Could you check a few things on this model? Use its own coordinates, in mm. A direction names the side the tool comes from. Coordinates: 2 decimals unless noted, no trailing zeros. Order: outer loops, then holes, each group sorted by start corner. A loop starts at its lowest first (then second) coordinate and runs counter-clockwise, first axis right, second up. Notation, with made-up numbers: (58, 53) -> (97, 53) arc R18 cw to (97, 84) -> close; hole circle Ø4 at (0, -14). An arc over 180 degrees is marked (long way). Return JSON: item names as keys, results as strings. Group by question number.
Autodesk Inventor part; units mm, degrees
ref_plane "YZ Plane" through (0, 0, 0) normal (1, 0, 0) x (0, 1, 0)
ref_plane "XZ Plane" through (0, 0, 0) normal (0, 1, 0) x (-1, 0, 0)
ref_plane "XY Plane" through (0, 0, 0) normal (0, 0, 1) x (1, 0, 0)
sketch "Sketch1" plane through (0, 0, 0) normal (0, 0, 1) x (1, 0, 0)
  line L0 (-20, 22.5) -> (20, 22.5)
  line L1 (20, 22.5) -> (20, -100)
  line L2 (20, -100) -> (-20, -100)
  line L3 (-20, -100) -> (-20, 22.5)
  circle A0 centre (0, 0) radius 2.5
  dimension "d0" = 122.5
  dimension "d1" = 40
  dimension "d2" = 20
  dimension "d3" = 22.5
  dimension "d4" = 5
extrude "Extrusion1" add sketch "Sketch1" along normal blind 5
sketch "Sketch2" plane through (0, 0, 5) normal (0, 0, 1) x (1, 0, 0)
  line L0 (20, 22.5) -> (-20, 22.5)
  line L1 (-20, -100) -> (20, -100)
  line L2 (-20, 22.5) -> (20, 22.5)
  line L3 (20, 22.5) -> (20, -100)
  line L4 (20, -100) -> (-20, -100)
  line L5 (-20, -100) -> (-20, 22.5)
  line L6 (15, -95) -> (-15, -95)
  line L7 (-15, -95) -> (-15, 17.5)
  line L8 (-15, 17.5) -> (15, 17.5)
  line L9 (15, 17.5) -> (15, -95)
  point P0 (0, 0)
  dimension "d7" = 5
  dimension "d8" = 5
  dimension "d9" = 5
  dimension "d10" = 5
extrude "Extrusion2" add sketch "Sketch2" along normal blind 35
sketch "Sketch3" plane through (-20, -100, 0) normal (0, -1, 0) x (1, 0, 0)
  circle A0 centre (20, 20) radius 8.5
  line L0 (40, 0) -> (40, 40)
  line L1 (0, 0) -> (40, 0)
  circle A1 centre (20, 11.5) radius 1.5
  circle A2 centre (20, 28.5) radius 1.5
  circle A3 centre (20, 20) radius 3.75
  line L2 (0, 0) -> (0, 40)
  point P0 (20, 0)
  dimension "d13" = 20
  dimension "d14" = 20
  dimension "d15" = 17
  dimension "d16" = 3
  dimension "d17" = 7.5
  dimension "d18" = 3
  dimension "d19" = 20
  dimension "d20" = 20
sketch "Sketch4" plane through (0, 0, 5) normal (0, 0, 1) x (1, 0, 0)
  line L0 (-15, 17.5) -> (-15, -95)
  line L1 (15, 17.5) -> (15, -95)
  line L2 (-15, 17.5) -> (15, 17.5)
  line L3 (15, 17.5) -> (15, -17.5)
  line L4 (15, -17.5) -> (-15, -17.5)
  line L5 (-15, -17.5) -> (-15, 17.5)
  point P0 (0, 0)
  point P1 (-15, -17.5)
  dimension "d21" = 35
extrude "Extrusion3" add sketch "Sketch4" along normal blind 20
sketch "Sketch5" plane through (0, 0, 0) normal (0, 0, -1) x (-1, 0, 0)
  circle A0 centre (0, 0) radius 2.5
  circle A1 centre (0, 0) radius 9.5
  dimension "d24" = 19
extrude "Extrusion4" cut sketch "Sketch5" against normal blind 12.5 contours A0 | A1
sketch "Sketch6" plane through (0, 0, 0) normal (0, 0, -1) x (-1, 0, 0)
  circle A0 centre (0, 0) radius 11.5
  dimension "d27" = 23
extrude "Extrusion5" cut sketch "Sketch6" against normal blind 6.5
fillet "Fillet1" radius 2 2 edges at (-20, 22.5, 20) (20, 22.5, 20)
sketch "Sketch7" plane through (0, 0, 0) normal (0, 0, -1) x (-1, 0, 0)
  circle A0 centre (0, 0) radius 6.2
  circle A1 centre (0, 6.2) radius 1.45
  line L0 (0, 6.2) -> (0, 0)
  line L1 (0, 0) -> (6.4707, -3.7359)
  line L2 (0, 0) -> (-6.6791, -3.8562)
  circle A2 centre (5.3694, -3.1) radius 1.45
  circle A3 centre (-5.3694, -3.1) radius 1.45
  dimension "d31" = 12.4
  dimension "d32" = 120
  dimension "d33" = 120
  dimension "d34" = 2.9
  dimension "d35" = 2.9
  dimension "d36" = 2.9
extrude "Extrusion6" cut sketch "Sketch7" against normal blind 25 contours A1 L0 A0 | A0 A1 | A2 A0 | A0 L1 A2 | L0 A1 A0 | A0 A2 L1 | A3 L2 A0 | A0 L2 A3 | A3 A0 L2 | A3 L2 A0
sketch "Sketch8" plane through (0, 0, 25) normal (0, 0, 1) x (1, 0, 0)
  circle A0 centre (5.3694, -3.1) radius 1.45
  circle A1 centre (5.3694, -3.1) radius 4
  circle A2 centre (-5.3694, -3.1) radius 1.45
  circle A3 centre (-5.3694, -3.1) radius 4
  circle A4 centre (0, 6.2) radius 1.45
  circle A5 centre (0, 6.2) radius 4
  point P0 (0, 0)
  dimension "d39" = 8
  dimension "d40" = 8
  dimension "d41" = 8
extrude "Extrusion7" cut sketch "Sketch8" against normal blind 7
fillet "Fillet2" radius 2 3 edges at (0, -17.5, 5) (-15, -56.25, 5) (15, -56.25, 5)
sketch "Sketch9" plane through (0, 0, 40) normal (0, 0, 1) x (1, 0, 0)
  line L0 (20, -100) -> (20, 20.5)
  line L1 (-20, 20.5) -> (-20, -100)
  line L2 (20, -100) -> (-20, -100)
  line L3 (-20, -100) -> (-20, -60)
  line L4 (-20, -60) -> (20, -60)
  line L5 (20, -60) -> (20, -100)
  line L6 (0, -60) -> (-20, -60)
  line L7 (-20, -60) -> (-20, -100)
  line L8 (-20, -100) -> (0, -100)
  line L9 (0, -100) -> (0, -60)
  line L10 (15, -95) -> (-15, -95)
  line L11 (15, -65) -> (-15, -65)
  line L12 (-15, -65) -> (-15, -95)
  line L13 (-15, -95) -> (15, -95)
  line L14 (15, -95) -> (15, -65)
  point P0 (0, 0)
  dimension "d45" = 40
  dimension "d46" = 5
  dimension "d47" = 5
extrude "Extrusion8" add sketch "Sketch9" along normal blind 60 contours L2 L9 L10 L14 L11 L4 L0 | L2 L1 L4 L9 L11 L12 L10
sketch "Sketch10" plane through (0, 0, 100) normal (0, 0, 1) x (1, 0, 0)
  line L0 (-20, -100) -> (20, -100)
  line L1 (20, -100) -> (20, 20.5)
  line L2 (-20, -100) -> (20, -100)
  line L3 (20, -100) -> (20, -60)
  line L4 (20, -60) -> (-20, -60)
  line L5 (-20, -60) -> (-20, -100)
  point P0 (0, 0)
  dimension "d50" = 40
extrude "Extrusion9" add sketch "Sketch10" against normal blind 5
sketch "Sketch11" plane through (0, 0, 100) normal (0, 0, 1) x (1, 0, 0)
  circle A0 centre (0, -80) radius 8.5
  line L0 (20, -100) -> (20, -60)
  line L1 (-20, -100) -> (20, -100)
  circle A1 centre (0, -71.5) radius 1.5
  circle A2 centre (0, -88.5) radius 1.5
  line L2 (-20, -60) -> (-20, -100)
  circle A3 centre (0, -80) radius 4
  point P0 (0, 0)
  dimension "d53" = 20
  dimension "d54" = 20
  dimension "d55" = 17
  dimension "d56" = 3
  dimension "d57" = 3
  dimension "d58" = 20
  dimension "d59" = 20
  dimension "d62" = 8
extrude "Extrusion10" cut sketch "Sketch11" against normal blind 5 contours A1 A0 | A0 A1 | A2 A0 | A0 A2 | A3
sketch "Sketch12" plane through (-15, -60, 40) normal (0, 1, 0) x (1, 0, 0)
  line L0 (0, 0) -> (30, 0)
  line L1 (0, 0) -> (30, 0)
  line L2 (30, 0) -> (30, -55)
  line L3 (30, -55) -> (0, -55)
  line L4 (0, -55) -> (0, 0)
  point P0 (15, 40)
extrude "Extrusion11" cut sketch "Sketch12" against normal blind 5
sketch "Sketch13" plane through (0, 0, 40) normal (0, 0, 1) x (1, 0, 0)
  line L0 (-20, 20.5) -> (-20, -100)
  line L1 (20, -60) -> (20, 20.5)
  line L2 (-20, -21.5352) -> (20, -21.5352)
  line L3 (20, -21.5352) -> (20, -29.5352)
  line L4 (20, -29.5352) -> (-20, -29.5352)
  line L5 (-20, -29.5352) -> (-20, -21.5352)
  line L6 (20, -37.5352) -> (-20, -37.5352)
  line L7 (-20, -37.5352) -> (-20, -45.5352)
  line L8 (-20, -45.5352) -> (20, -45.5352)
  line L9 (20, -45.5352) -> (20, -37.5352)
  point P0 (0, 0)
  point P1 (-20, -37.5352)
  point P2 (-20, -29.5352)
  point P3 (20, -21.5352)
  dimension "d65" = 8
  dimension "d66" = 8
  dimension "d67" = 8
extrude "Extrusion12" add sketch "Sketch13" against normal blind 5 contours L2 L1 L4 L0 | L6 L1 L8 L0
fillet "Fillet3" radius 3 4 edges at (15, -29.5352, 37.5) (15, -37.5352, 37.5) (-15, -29.5352, 37.5) (-15, -37.5352, 37.5)
sketch "Sketch14" plane through (0, 0, 95) normal (0, 0, -1) x (-1, 0, 0)
  line L0 (15, -95) -> (-15, -95)
  line L1 (-15, -95) -> (15, -95)
  line L2 (15, -95) -> (15, -60)
  line L3 (15, -60) -> (-15, -60)
  line L4 (-15, -60) -> (-15, -95)
  circle A0 centre (0, -80) radius 4
  circle A1 centre (0, -80) radius 4
  circle A2 centre (0, -71.5) radius 1.5
  circle A3 centre (0, -71.5) radius 1.5
  circle A4 centre (0, -88.5) radius 1.5
  circle A5 centre (0, -88.5) radius 1.5
  point P0 (0, 0)
extrude "Extrusion13" add sketch "Sketch14" along normal blind 3
sketch "Sketch15" plane through (0, 0, 92) normal (0, 0, -1) x (-1, 0, 0)
  circle A0 centre (0, -80) radius 4
  circle A1 centre (0, -80) radius 13
  point P0 (0, 0)
  dimension "d73" = 26
extrude "Extrusion14" cut sketch "Sketch15" against normal blind 4 contours A0 | A1
fillet "Fillet4" radius 3 5 edges at (-20, -80, 100) (20, -80, 100) (-17.5, -60, 40) (17.5, -60, 40) (0, -100, 0)
properties part number "Link4_v2"
Q1. I need wall thicknesses on line 1 along Y through (x, z) = (0, 14.25); line 2 along Y through (x, z) = (0, 21.25); line 3 along Y through (x, z) = (2.5, 34). Which ranges of each line are inside material? Lowest first, please. Write a range as from..to.
Q2. On a 3-axis mill with a long thin cutter (end or side, diameter ignored), from which of +Z, -Z, +X, -X, +Y, -Y can I reach the whole of each face in a straight line? I mean faces 4 (the flat face through (15, -50, 39)), 5 (the cylindrical face through (-14.145, -36.633, 37.535)), 6 (the cylindrical face through (-6.75, -2.66, 15.21)). Say none if no direction works.
Q3. I want a section at B-B on z = 27.5. Please give me the cut outline in (x, y), and give its area (3 significant figures).
Q4. I want a section at A-A on z = 16.5. Please give me the cut outline in (x, y), and give its area (3 significant figures).
Q5. I'm going to push flat-ended pins straight in: pin 1 Ø6 at (x, y) = (10, -47) entering from +Z; pin 2 Ø5 at (x, z) = (-7, 73) entering from +Y; pin 3 Ø5 at (x, y) = (6, -14) entering from -Z; pin 4 Ø2.5 at (x, y) = (-5.37, -3.1) entering from -Z. Where does each tip first touch, or does it pass through?
Q6. I want a section at D-D on y = 6.2. Please give me the cut outline in (x, z).
Q7. I want a section at C-C on y = -44. Please give me the cut outline in (x, z).
Q8. We'd pull the mould along Z, two halves only. Please class faces 1 (the cylindrical face through (1.5, 11.4, 3.2)), 2 (the flat face through (0, -57, 5)), 3 (the flat face through (0, -36, 0)): pulls with the +Z half, pulls with the -Z half, needs draft (parallel to the pull), parting line crosses it, or undercut.
Response values:
{
 "1": {"line 1": "y = -100..-95, -17.5..4.75, 7.65..22.5", "line 2": "y = -100..-95, -17.5..2.2, 10.2..22.5", "line 3": "y = -100..-95, 17.5..22.5"},
 "2": {"face 4": "none", "face 5": "+Z", "face 6": "+Z, -Z"},
 "3": {"outline": "(-20, -100) -> (20, -100) -> (20, 20.5) arc R2 ccw to (18, 22.5) -> (-18, 22.5) arc R2 ccw to (-20, 20.5) -> close; hole (-15, -95) -> (15, -95) -> (15, 17.5) -> (-15, 17.5) -> close", "area": "1,520 mm²"},
 "4": {"outline": "(-20, -100) -> (20, -100) -> (20, 20.5) arc R2 ccw to (18, 22.5) -> (-18, 22.5) arc R2 ccw to (-20, 20.5) -> close; hole (-15, -95) -> (15, -95) -> (15, -17.5) -> (-15, -17.5) -> close; hole circle Ø2.9 at (-5.37, -3.1); hole circle Ø2.9 at (0, 6.2); hole circle Ø2.9 at (5.37, -3.1)", "area": "2,550 mm²"},
 "5": {"pin 1": "stops at z = 40", "pin 2": "stops at y = -95", "pin 3": "stops at z = 0", "pin 4": "passes through"},
 "6": {"outline": "(-20, 0) -> (-9.69, 0) -> (-9.69, 6.5) -> (-7.2, 6.5) -> (-7.2, 12.5) -> (-1.45, 12.5) -> (-1.45, 18) -> (-4, 18) -> (-4, 25) -> (-15, 25) -> (-15, 40) -> (-20, 40) -> close; (1.45, 12.5) -> (7.2, 12.5) -> (7.2, 6.5) -> (9.69, 6.5) -> (9.69, 0) -> (20, 0) -> (20, 40) -> (15, 40) -> (15, 25) -> (4, 25) -> (4, 18) -> (1.45, 18) -> close"},
 "7": {"outline": "(-20, 0) -> (20, 0) -> (20, 40) -> (-20, 40) -> close; hole (-15, 7) arc R2 ccw to (-13, 5) -> (13, 5) arc R2 ccw to (15, 7) -> (15, 35) -> (-15, 35) -> close"},
 "8": {"face 1": "needs draft", "face 2": "undercut", "face 3": "pulls with the -Z half"}
}
